Autodesk Inventor part; units mm, degrees
ref_plane "YZ Plane" through (0, 0, 0) normal (1, 0, 0) x (0, 1, 0)
ref_plane "XZ Plane" through (0, 0, 0) normal (0, 1, 0) x (-1, 0, 0)
ref_plane "XY Plane" through (0, 0, 0) normal (0, 0, 1) x (1, 0, 0)
sketch "Sketch1" plane through (0, 0, 0) normal (0, 1, 0) x (-1, 0, 0)
  line L0 (0, 0) -> (0, 50.8)
  line L1 (0, 50.8) -> (25.4, 50.8)
  line L2 (25.4, 50.8) -> (25.4, 0)
  line L3 (25.4, 0) -> (0, 0)
  circle A0 centre (12.7, 38.1) radius 3.302
  circle A1 centre (12.7, 12.7) radius 3.302
  line L4 (0, 25.4) -> (25.4, 25.4) construction
  line L5 (12.7, 38.1) -> (12.7, 12.7) construction
  point P0 (12.7, 25.4)
  dimension "d0" = 50.8
  dimension "d1" = 25.4
  dimension "d2" = 6.604
  dimension "d3" = 6.604
  dimension "d4" = 25.4
extrude "Extrusion1" add sketch "Sketch1" along normal blind 3.175
fillet "Fillet1" radius 1.5875 4 edges at (-25.4, 1.5875, 50.8) (0, 1.5875, 50.8) (0, 1.5875, 0) (-25.4, 1.5875, 0)
equation "\"d3\" = d2"
properties part number "Chassis Connector Plate V1.500" material "Aluminum 6061"
Geometry: final body of the model. Coordinates: model frame, mm. Coordinates: 2 decimals unless noted, no trailing zeros. Order: outer loops, then holes, each group sorted by start corner. A loop starts at its lowest first (then second) coordinate and runs counter-clockwise, first axis right, second up.
(1) First-contact query: pin 1 (5.5 mm diameter, centred on x = -12.7, z = 38.1, fed in from -Y). Flat tip, straight axial feed; report the tip coordinate or a pass-through.
(2) Section query B-B (x = -12.7). Return the cut outline in (y, z) (3 decimals), plus the area to 3 significant figures.
(3) Material intervals for probe 1 along Z at (x, y) = (-12.7, 1.85); probe 2 along X at (y, z) = (1.5, 38); probe 3 along Z at (x, y) = (-10, 2.45), sorted ascending.
(4) Section query A-A (z = 38.1). Return the cut outline in (x, y) (3 decimals).
(5) Section query C-C (y = 2.15). Return the cut outline in (x, z) (1 decimal), plus the area to 3 significant figures.
(6) Draft query along X for faces 1 (the face through (-15.85, 1.57, 37.11)), 2 (the face through (-24.92, 1.61, 0.45)), 3 (the face through (-0.48, 1.61, 50.35)). Return one class per face: pulls with the +X half, pulls with the -X half, needs draft (parallel to the pull), parting line crosses it, or undercut.
Solution:
1. pin 1: passes through
2. outline: (0, 0) - (3.175, 0) - (3.175, 9.398) - (0, 9.398) - close; (0, 16.002) - (3.175, 16.002) - (3.175, 34.798) - (0, 34.798) - close; (0, 41.402) - (3.175, 41.402) - (3.175, 50.8) - (0, 50.8) - close
2. area: 119 mm2
3. probe 1: z = 0 to 9.4, 16 to 34.8, 41.4 to 50.8
3. probe 2: x = -25.4 to -16, -9.4 to 0
3. probe 3: z = 0 to 10.8, 14.6 to 36.2, 40 to 50.8
4. outline: (-25.4, 0) - (-16.002, 0) - (-16.002, 3.175) - (-25.4, 3.175) - close; (-9.398, 0) - (0, 0) - (0, 3.175) - (-9.398, 3.175) - close
5. outline: (-25.4, 1.6) arc R1.6 ccw to (-23.8, 0) - (-1.6, 0) arc R1.6 ccw to (0, 1.6) - (0, 49.2) arc R1.6 ccw to (-1.6, 50.8) - (-23.8, 50.8) arc R1.6 ccw to (-25.4, 49.2) - close; hole circle Ø6.6 at (-12.7, 12.7); hole circle Ø6.6 at (-12.7, 38.1)
5. area: 1,220 mm2
6. face 1: undercut
6. face 2: pulls with the -X half
6. face 3: pulls with the +X half
